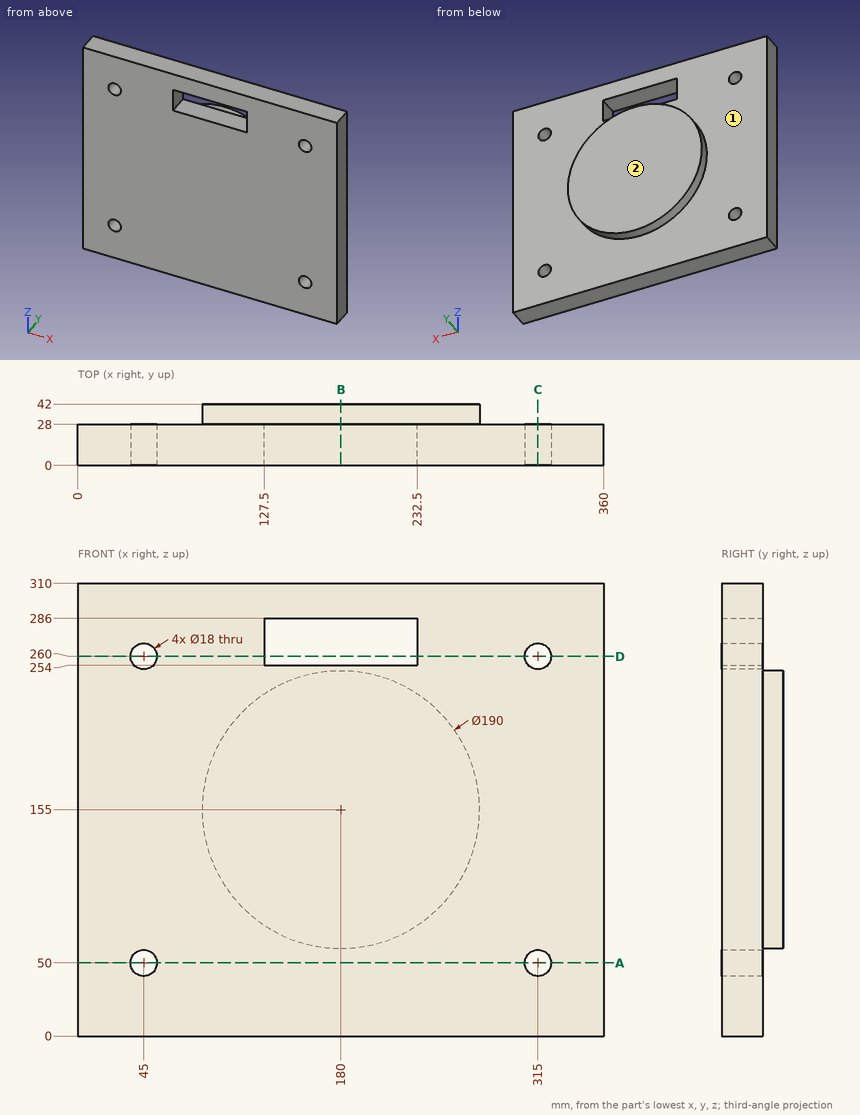
Input: dimensioned drawing with shaded views. Units: mm. Origin: part minimum x, y, z. A direction names the side the tool comes from. Round coordinates to 2 decimals unless told otherwise and drop trailing zeros. Loops run counter-clockwise (first coordinate to the right, second up) from the corner with the lowest first, then second, coordinate; pieces in that order, holes last. Notation, with made-up numbers: M -30.5,2 L 26.5,2 A20 cw 26.5,38 Z; hole C -38,20 d4. An arc over 180 degrees is marked long. Return JSON: item names as keys, results as strings. Group by question number.
1. Section query D-D on z = 260. Output: boundary loops of the cut face in (x, y).
2. Pin query (flat end, axial travel): pin 1 (4 mm diameter, centred on x = 271, z = 130, fed in from -Y); pin 2 (10 mm diameter, centred on x = 105, z = 227, fed in from +Y). Return the tip coordinate at first contact, or that it passes through.
3. Section query B-B on x = 180. Output: boundary loops of the cut face in (y, z), and give its area (3 significant figures).
4. Section query A-A on z = 50. Output: boundary loops of the cut face in (x, y), and give its area (3 significant figures).
5. Reachability of the marked faces 1 and 2 from +Z, -Z, +X, -X, +Y, -Y: full face, straight path, thin tool, end or side. Return the list, or none.
6. Section query C-C on x = 315. Output: boundary loops of the cut face in (y, z), and give its area (3 significant figures).
7. Material intervals for line 1 along X through (y, z) = (13.5, 50); line 2 along Z through (x, y) = (315, 13); line 3 along X through (y, z) = (11, 260), sorted ascending. Write a range as from..to.
Checks:
{
 "1": {"outline": "M 0,0 L 36,0 L 36,28 L 0,28 Z; M 54,0 L 127.5,0 L 127.5,28 L 54,28 Z; M 232.5,0 L 306,0 L 306,28 L 232.5,28 Z; M 324,0 L 360,0 L 360,28 L 324,28 Z"},
 "2": {"pin 1": "stops at y = 0", "pin 2": "stops at y = 28"},
 "3": {"outline": "M 0,0 L 28,0 L 28,60 L 42,60 L 42,250 L 28,250 L 28,254 L 0,254 Z; M 0,286 L 28,286 L 28,310 L 0,310 Z", "area": "10,400 mm²"},
 "4": {"outline": "M 0,0 L 36,0 L 36,28 L 0,28 Z; M 54,0 L 306,0 L 306,28 L 54,28 Z; M 324,0 L 360,0 L 360,28 L 324,28 Z", "area": "9,070 mm²"},
 "5": {"face 1": "+Y", "face 2": "+Z, -Z, +X, -X, +Y"},
 "6": {"outline": "M 0,0 L 28,0 L 28,41 L 0,41 Z; M 0,59 L 28,59 L 28,251 L 0,251 Z; M 0,269 L 28,269 L 28,310 L 0,310 Z", "area": "7,670 mm²"},
 "7": {"line 1": "x = 0..36, 54..306, 324..360", "line 2": "z = 0..41, 59..251, 269..310", "line 3": "x = 0..36, 54..127.5, 232.5..306, 324..360"}
}
